```python
from build123d import *

# Parameters (mm, degrees)
SKETCH_1_W          = 85
SKETCH_1_H          = 75
EXTRUDE_1_DEPTH     = 1.6
CUT_EXTRUDE_1_REACH = 58.701
SKETCH_2_R          = 1.65
SKETCH_8_W          = 85
SKETCH_8_H          = 25
EXTRUDE_3_DEPTH     = 1.6
CHAMFER_2_SIZE      = 3
CHAMFER_3_SIZE      = 20
CUT_EXTRUDE_4_REACH = 77.598
CUT_EXTRUDE_5_REACH = 77.598
SKETCH_9_R          = 1.65


with BuildPart() as part:
    # 草图1 → 凸台-拉伸1 (new body)
    with BuildSketch(Plane(origin=(0, 0, 0), x_dir=(1, 0, 0), z_dir=(0, 1, 0))):
        Rectangle(SKETCH_1_W, SKETCH_1_H)
    extrude(amount=EXTRUDE_1_DEPTH)

    # 草图2 → 切除-拉伸1 (cut, up to next)
    with BuildSketch(Plane(origin=(0, 1.6, 0), x_dir=(1, 0, 0), z_dir=(0, 1, 0)), mode=Mode.PRIVATE) as cut_extrude_1_sk1:
        with Locations(Location((-28, 20, 0), (0, 0, 270))):
            Circle(SKETCH_2_R)
    cut_extrude_1_tool1 = extrude(cut_extrude_1_sk1.sketch, amount=-CUT_EXTRUDE_1_REACH, mode=Mode.PRIVATE) & part.part
    # 草图2 → 切除-拉伸1 (cut, up to next)
    with BuildSketch(Plane(origin=(0, 1.6, 0), x_dir=(1, 0, 0), z_dir=(0, 1, 0)), mode=Mode.PRIVATE) as cut_extrude_1_sk2:
        with Locations(Location((-28, -20, 0), (0, 0, 270))):
            Circle(SKETCH_2_R)
    cut_extrude_1_tool2 = extrude(cut_extrude_1_sk2.sketch, amount=-CUT_EXTRUDE_1_REACH, mode=Mode.PRIVATE) & part.part
    # 草图2 → 切除-拉伸1 (cut, up to next)
    with BuildSketch(Plane(origin=(0, 1.6, 0), x_dir=(1, 0, 0), z_dir=(0, 1, 0)), mode=Mode.PRIVATE) as cut_extrude_1_sk3:
        with Locations(Location((28, 20, 0), (0, 0, 270))):
            Circle(SKETCH_2_R)
    cut_extrude_1_tool3 = extrude(cut_extrude_1_sk3.sketch, amount=-CUT_EXTRUDE_1_REACH, mode=Mode.PRIVATE) & part.part
    # 草图2 → 切除-拉伸1 (cut, up to next)
    with BuildSketch(Plane(origin=(0, 1.6, 0), x_dir=(1, 0, 0), z_dir=(0, 1, 0)), mode=Mode.PRIVATE) as cut_extrude_1_sk4:
        with Locations(Location((28, -20, 0), (0, 0, 270))):
            Circle(SKETCH_2_R)
    cut_extrude_1_tool4 = extrude(cut_extrude_1_sk4.sketch, amount=-CUT_EXTRUDE_1_REACH, mode=Mode.PRIVATE) & part.part
    add(cut_extrude_1_tool1.solids().sort_by_distance((-28, 1.6, -20))[0], mode=Mode.SUBTRACT)
    add(cut_extrude_1_tool2.solids().sort_by_distance((-28, 1.6, 20))[0], mode=Mode.SUBTRACT)
    add(cut_extrude_1_tool3.solids().sort_by_distance((28, 1.6, -20))[0], mode=Mode.SUBTRACT)
    add(cut_extrude_1_tool4.solids().sort_by_distance((28, 1.6, 20))[0], mode=Mode.SUBTRACT)

    # 草图8 → 凸台-拉伸3 (add)
    with BuildSketch(Plane(origin=(0, 0, 0), x_dir=(1, 0, 0), z_dir=(0, 1, 0))):
        with Locations((0, 50)):
            Rectangle(SKETCH_8_W, SKETCH_8_H)
    extrude(amount=EXTRUDE_3_DEPTH)

    # 倒角2
    chamfer_2_edges = [part.edges().sort_by_distance(p)[0] for p in [
        (42.5, 0.8, -62.5),
        (-42.5, 0.8, -62.5),
    ]]
    chamfer(chamfer_2_edges, length=CHAMFER_2_SIZE)

    # 倒角3
    chamfer_3_edges = [part.edges().sort_by_distance(p)[0] for p in [
        (42.5, 0.8, 37.5),
        (-42.5, 0.8, 37.5),
    ]]
    chamfer(chamfer_3_edges, length=CHAMFER_3_SIZE)

    # 草图7 → 切除-拉伸4 (cut, up to next)
    with BuildSketch(Plane(origin=(0, 1.6, 0), x_dir=(1, 0, 0), z_dir=(0, 1, 0)), mode=Mode.PRIVATE) as cut_extrude_4_sk1:
        Polygon((-35, -25), (-35, -20), (-42.5, -12.5), (-42.5, -17.5), align=None)
    cut_extrude_4_tool1 = extrude(cut_extrude_4_sk1.sketch, amount=-CUT_EXTRUDE_4_REACH, mode=Mode.PRIVATE) & part.part
    cut_extrude_4 = cut_extrude_4_tool1.solids().sort_by_distance((-38.75, 1.6, 18.75))[0]
    add(cut_extrude_4, mode=Mode.SUBTRACT)

    # 镜向1: 切除-拉伸4 across plane
    add(cut_extrude_4.mirror(Plane(origin=(0, 0, 0), x_dir=(0, 0, 1), z_dir=(1, 0, 0))), mode=Mode.SUBTRACT)

    # 草图9 → 切除-拉伸5 (cut, up to next)
    with BuildSketch(Plane(origin=(0, 1.6, 0), x_dir=(1, 0, 0), z_dir=(0, 1, 0)), mode=Mode.PRIVATE) as cut_extrude_5_sk1:
        with Locations(Location((-28, 55.75, 0), (0, 0, 270))):
            Circle(SKETCH_9_R)
    cut_extrude_5_tool1 = extrude(cut_extrude_5_sk1.sketch, amount=-CUT_EXTRUDE_5_REACH, mode=Mode.PRIVATE) & part.part
    # 草图9 → 切除-拉伸5 (cut, up to next)
    with BuildSketch(Plane(origin=(0, 1.6, 0), x_dir=(1, 0, 0), z_dir=(0, 1, 0)), mode=Mode.PRIVATE) as cut_extrude_5_sk2:
        with Locations(Location((-28, 45.75, 0), (0, 0, 270))):
            Circle(SKETCH_9_R)
    cut_extrude_5_tool2 = extrude(cut_extrude_5_sk2.sketch, amount=-CUT_EXTRUDE_5_REACH, mode=Mode.PRIVATE) & part.part
    # 草图9 → 切除-拉伸5 (cut, up to next)
    with BuildSketch(Plane(origin=(0, 1.6, 0), x_dir=(1, 0, 0), z_dir=(0, 1, 0)), mode=Mode.PRIVATE) as cut_extrude_5_sk3:
        with Locations(Location((28, 55.75, 0), (0, 0, 270))):
            Circle(SKETCH_9_R)
    cut_extrude_5_tool3 = extrude(cut_extrude_5_sk3.sketch, amount=-CUT_EXTRUDE_5_REACH, mode=Mode.PRIVATE) & part.part
    # 草图9 → 切除-拉伸5 (cut, up to next)
    with BuildSketch(Plane(origin=(0, 1.6, 0), x_dir=(1, 0, 0), z_dir=(0, 1, 0)), mode=Mode.PRIVATE) as cut_extrude_5_sk4:
        with Locations(Location((28, 45.75, 0), (0, 0, 270))):
            Circle(SKETCH_9_R)
    cut_extrude_5_tool4 = extrude(cut_extrude_5_sk4.sketch, amount=-CUT_EXTRUDE_5_REACH, mode=Mode.PRIVATE) & part.part
    add(cut_extrude_5_tool1.solids().sort_by_distance((-28, 1.6, -55.75))[0], mode=Mode.SUBTRACT)
    add(cut_extrude_5_tool2.solids().sort_by_distance((-28, 1.6, -45.75))[0], mode=Mode.SUBTRACT)
    add(cut_extrude_5_tool3.solids().sort_by_distance((28, 1.6, -55.75))[0], mode=Mode.SUBTRACT)
    add(cut_extrude_5_tool4.solids().sort_by_distance((28, 1.6, -45.75))[0], mode=Mode.SUBTRACT)


solid = part.part
```
Model file for the job. Use its own axes, mm. Give positions to 0.01 mm unless a question says otherwise; leave off trailing zeros. Loops run counter-clockwise (first coordinate to the right, second up) from the corner with the lowest first, then second, coordinate; pieces in that order, holes last. Notation, with made-up numbers: (69.5, 68) -> (118.5, 68) arc R5 cw to (118.5, 75) -> close; hole circle Ø11 at (59.25, 14.5). An arc over 180 degrees is marked (long way). Use CSV: the item, a comma, the result in double quotes. Start each with the question number.
1) Flat gauge pin, fed straight in: pin 1 Ø0.5 at (y, z) = (0.5, 21.5) entering from -X. Where does the tip first touch, or does it go through?
2) Mould opens along X. For faces 1 (the cylindrical face through (29.636, 0.811, -45.965)), 2 (the cylindrical face through (-26.364, 0.811, -20.215)), 3 (the flat face through (-29, 1, 31)), 4 (the flat face through (-1, 1.6, -13)) say: released by +X, released by -X, zero draft, split by the parting line, or undercut.
3) Slice it at A-A on x = 28. Give the cut face in (y, z), plus the area to 3 significant figures.
4) Slice it at B-B on y = 0.3. Give the number of separate pieces and of enclosed holes in the cut face, plus the area to 3 significant figures.
5) Slice it at C-C on z = -55.75. Give the cut face in (x, y), plus the area to 3 significant figures.
6) Wall check: line 1 (X direction, y = 0.35, z = -46); line 2 (X direction, y = 1.1, z = 20); line 3 (Z direction, x = -27, y = 1.55). Give the ranges that are in metal, low to high.
7) Slice it at D-D on z = 27. Give the cut face in (x, y), plus the area to 3 significant figures.
Computed values:
1,pin 1,"stops at x = -35"
2,face 1,"undercut"
2,face 2,"undercut"
2,face 3,"released by -X"
2,face 4,"zero draft"
3,outline,"(0, -62.5) -> (1.6, -62.5) -> (1.6, -57.4) -> (0, -57.4) -> close; (0, -54.1) -> (1.6, -54.1) -> (1.6, -47.4) -> (0, -47.4) -> close; (0, -44.1) -> (1.6, -44.1) -> (1.6, -21.65) -> (0, -21.65) -> close; (0, -18.35) -> (1.6, -18.35) -> (1.6, 18.35) -> (0, 18.35) -> close; (0, 21.65) -> (1.6, 21.65) -> (1.6, 32) -> (0, 32) -> close"
3,area,"130 mm^2"
4,separate pieces,"1"
4,enclosed holes,"8"
4,area,"7,950 mm^2"
5,outline,"(-42.5, 0) -> (-29.65, 0) -> (-29.65, 1.6) -> (-42.5, 1.6) -> close; (-26.35, 0) -> (26.35, 0) -> (26.35, 1.6) -> (-26.35, 1.6) -> close; (29.65, 0) -> (42.5, 0) -> (42.5, 1.6) -> (29.65, 1.6) -> close"
5,area,"125 mm^2"
6,line 1,"x = -42.5 to -29.63, -26.37 to 26.37, 29.63 to 42.5"
6,line 2,"x = -35 to -29.65, -26.35 to 26.35, 29.65 to 35"
6,line 3,"z = -62.5 to -57.06, -54.44 to -47.06, -44.44 to -21.31, -18.69 to 18.69, 21.31 to 33"
7,outline,"(-33, 0) -> (33, 0) -> (33, 1.6) -> (-33, 1.6) -> close"
7,area,"106 mm^2"
